The figure shows three views and two pictorial views of one solid part (mm, origin at its lowest corner). Answer the questions. A direction names the side the tool comes from. Coordinates: 2 decimals unless noted, no trailing zeros. Write each loop counter-clockwise with the first axis right and the second up, starting at its lowest first coordinate (ties: lowest second). Pieces come first, ordered by that corner, then holes. Notation, with made-up numbers: (52, 70) - (77, 70) arc R13 cw to (77, 76) - close; hole circle Ø2 at (-5, 13.25). An arc over 180 degrees is marked (long way). Use a Markdown table: item, result. Add a question column.
(1) The part is cut by section C-C, the plane z = 78. Give the vertices of the cut face in (x, y), then the cut area to 3 significant figures.
(2) The part is cut by section A-A, the plane y = 626. Give the vertices of the cut face in (x, z), then the cut area to 3 significant figures.
(3) Find the intervals of material crossed by line 1 (Z direction, x = 139, y = 1636); line 2 (X direction, y = 1382.5, z = 110.5); line 3 (Y direction, x = 152, z = 134.5), in increasing order. Write a range as from..to.
(4) A tool of negligible diameter and unlimited length cuts with its end or side. For the marked faces 1 and 2, from which of +Z, -Z, +X, -X, +Y, -Y can it reach the whole face along a straight path? Write none if from no direction.
(5) Given pin 1 Ø2 at (y, z) = (1271, 32) entering from -X; pin 2 Ø3 at (x, z) = (41, 134) entering from -Y; pin 3 Ø1.5 at (x, y) = (279, 981) entering from -Z, each flat-ended and moving along its own axis, determine where each tip first touches the part or whether it passes through.
(6) The part is cut by section B-B, the plane x = 133. Give the vertices of the cut face in (y, z).
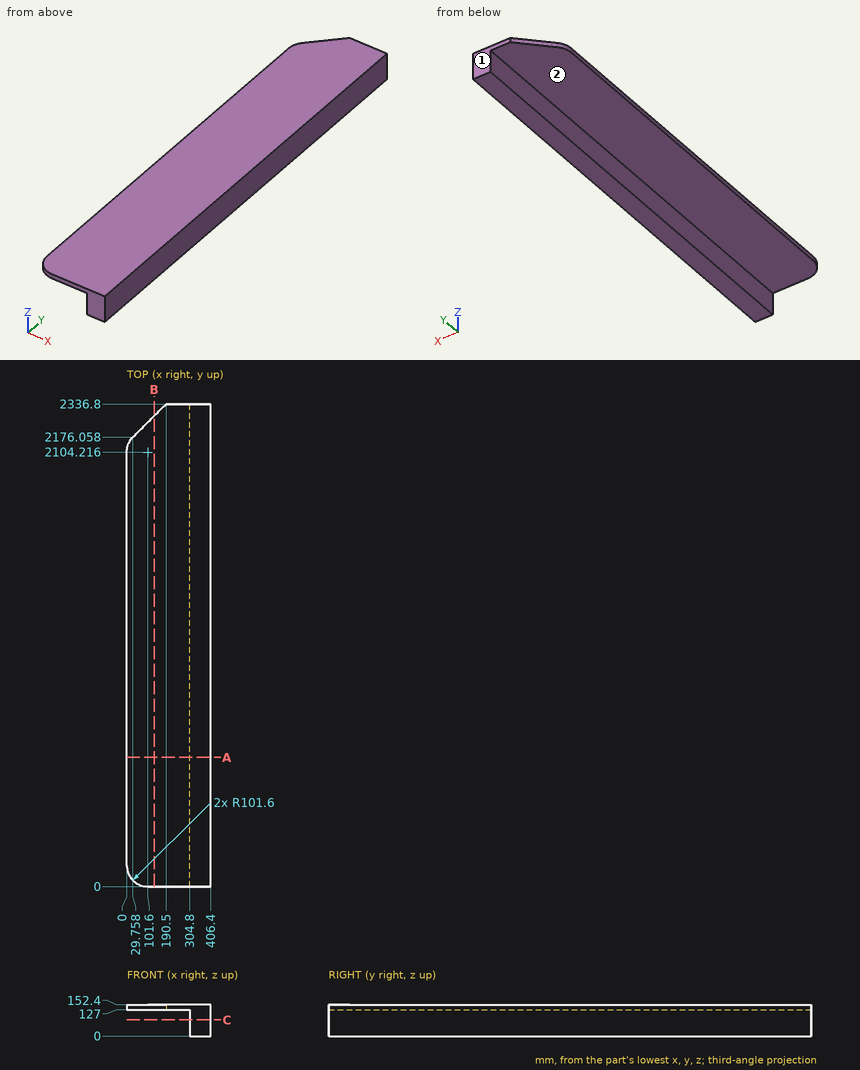
Model answer:
| question | item | result |
|---|---|---|
| 1 | outline | (304.8, 0) - (406.4, 0) - (406.4, 2336.8) - (304.8, 2336.8) - close |
| 1 | area | 237,000 mm^2 |
| 2 | outline | (0, 127) - (304.8, 127) - (304.8, 0) - (406.4, 0) - (406.4, 152.4) - (0, 152.4) - close |
| 2 | area | 23,200 mm^2 |
| 3 | line 1 | 127..152.4 |
| 3 | line 2 | 304.8..406.4 |
| 3 | line 3 | 0..2298.3 |
| 4 | face 1 | +Z, -Z, +X, -X, +Y |
| 4 | face 2 | -Z, -X, +Y, -Y |
| 5 | pin 1 | x = 304.8 |
| 5 | pin 2 | y = 18.96 |
| 5 | pin 3 | z = 127 |
| 6 | outline | (0, 127) - (2279.3, 127) - (2279.3, 152.4) - (0, 152.4) - close |
